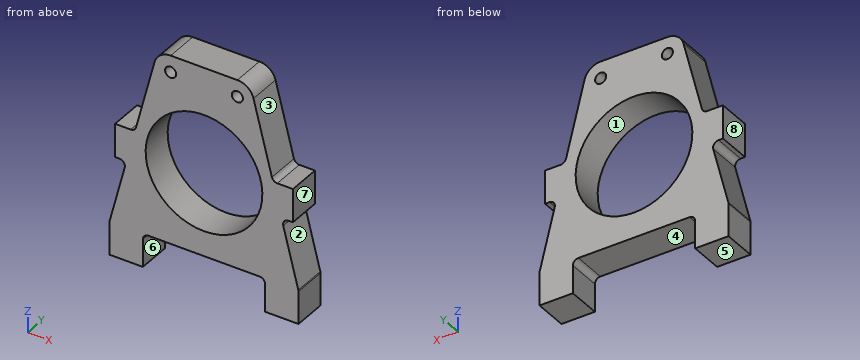
from build123d import *
from build123d import SkipClean  # not in build123d's __all__

# Parameters (mm, degrees)
F0_R     = 5
F1_DEPTH = 15
F2_R     = 5


with BuildPart() as f1:
    # F0 (on Front) → F1 (new body, symmetric)
    with BuildSketch(Plane.XZ):
        with BuildLine():
            Line((-85, 30), (-85, 0))
            Line((-85, 0), (-55, 0))
            Line((-55, 0), (-55, 30))
            Line((-55, 30), (0, 30))
            Line((0, 30), (0, 52.5))
            ThreePointArc((0, 52.5), (-52.5, 105), (0, 157.5))
            Line((0, 157.5), (0, 200))
            Line((0, 200), (-30, 200))
            ThreePointArc((-30, 200), (-39.2035469986, 196.8446073234), (-44.5349866907, 188.7059630193))
            Line((-44.5349866907, 188.7059630193), (-62.0528395496, 120))
            Line((-62.0528395496, 120), (-80, 120))
            Line((-80, 120), (-80, 90))
            Line((-80, 90), (-69.7018930331, 90))
            Line((-69.7018930331, 90), (-85, 30))
        make_face()
        with Locations((-30, 185)):
            Circle(F0_R, mode=Mode.SUBTRACT)
    extrude(amount=F1_DEPTH, both=True)

    # F2
    f2_edges = [f1.edges().sort_by_distance(p)[0] for p in [
        (-69.701893, 0, 90),
        (-62.05284, 0, 120),
        (-85, 0, 30),
        (-55, 0, 30),
    ]]
    fillet(f2_edges, radius=F2_R)

    # F3: F1 across plane


with BuildPart() as f1_1:
    add(f1.part, clean=False)
    with SkipClean():  # cleaning this boolean's faces spoils the solid; the shape is the same uncleaned
        add(f1.part.mirror(Plane.YZ), clean=False)


solid = f1_1.part
Source: CAD feature listing. Evaluate the final solid. Frame: model axes, mm. Face numbers are marked on the shaded views. A direction names the side the tool comes from. Give positions to 0.01 mm unless a question says otherwise; leave off trailing zeros. Order: outer loops, then holes, each group sorted by start corner. A loop starts at its lowest first (then second) coordinate and runs counter-clockwise, first axis right, second up. Notation, with made-up numbers: (33, 71.25) -> (92, 71.25) arc R32 cw to (92, 103.25) -> close; hole circle Ø1 at (-6, 18.5). An arc over 180 degrees is marked (long way). Write item = value, one per line.
Item 1: Section query B-B (x = 0). Output: boundary loops of the cut face in (y, z).
Check result:
outline = (-15, 30) -> (15, 30) -> (15, 52.5) -> (-15, 52.5) -> close; (-15, 157.5) -> (15, 157.5) -> (15, 200) -> (-15, 200) -> close
Item 2: Set-up query: the marked faces 5, 6, 7 and 8. Return all of +Z, -Z, +X, -X, +Y, -Y with unobstructed straight access to the full face (end or side cutting, diameter ignored); none if empty.
Check result:
face_5 = -Z, +X, -X, +Y, -Y
face_6 = -Z, +Y, -Y
face_7 = +Z, +X, +Y, -Y
face_8 = +Z, -X, +Y, -Y
Item 3: Section query A-A (z = 14.5). Output: boundary loops of the cut face in (x, y).
Check result:
outline = (-85, -15) -> (-55, -15) -> (-55, 15) -> (-85, 15) -> close; (55, -15) -> (85, -15) -> (85, 15) -> (55, 15) -> close
Item 4: Mould query, pull axis Z, two halves, no side actions, for the marked faces 1, 2, 3 and 4. Classes: +Z half, -Z half, draft (parallel to the pull), parting line (faces both ways), or undercut.
Check result:
face_1 = undercut
face_2 = undercut
face_3 = +Z half
face_4 = -Z half
Item 5: Contact query for flat-ended pins moving along their axis: pin 1 (8 mm diameter, centred on x = 42, y = 5.5, fed in from +Z); pin 2 (8 mm diameter, centred on y = 12, z = 164, fed in from -X); pin 3 (1.2 mm diameter, centred on x = -78.5, y = -2.5, fed in from -Z); pin 4 (15.5 mm diameter, centred on x = -75.5, y = 7, fed in from +Z). Output: stop coordinate, or through.
Check result:
pin_1 = 197.69
pin_2 = -51.85
pin_3 = 0
pin_4 = 120
Item 6: Section query D-D (z = 185). Output: boundary loops of the cut face in (x, y).
Check result:
outline = (-45.48, -15) -> (-35, -15) -> (-35, 15) -> (-45.48, 15) -> close; (-25, -15) -> (25, -15) -> (25, 15) -> (-25, 15) -> close; (35, -15) -> (45.48, -15) -> (45.48, 15) -> (35, 15) -> close
Item 7: Ray query, probe 1 along Z at (x, y) = (0, -5.25); probe 2 along Z at (x, y) = (30, 5.5); probe 3 along X at (y, z) = (-0.75, 182.5). Return the intervals inside material, ascending.
Check result:
probe_1 = 30 to 52.5, 157.5 to 200
probe_2 = 30 to 61.92, 148.08 to 180, 190 to 200
probe_3 = -46.12 to -34.33, -25.67 to 25.67, 34.33 to 46.12
Item 8: Section query C-C (y = -9.5). State how many separate pieces and enclosed holes the cut face has, then the cut area to 3 significant figures.
Check result:
separate_pieces = 1
enclosed_holes = 3
area = 15,300 mm²
